Design review of the part built by this model. Coordinates are the model's own, in mm. A direction names the side the tool comes from. Coordinates: 2 decimals unless noted, no trailing zeros. Write each loop counter-clockwise with the first axis right and the second up, starting at its lowest first coordinate (ties: lowest second). Pieces come first, ordered by that corner, then holes. Notation, with made-up numbers: (55.5, 13) - (60.5, 13) arc R19 cw to (60.5, 46) - close; hole circle Ø11 at (86.25, 11). An arc over 180 degrees is marked (long way). Use a Markdown table: item, result.
from build123d import *

# Parameters (mm, degrees)
SKETCH1_R           = 7
SKETCH1_R_2         = 2.75
BOSS_EXTRUDE1_DEPTH = 7
SKETCH2_R           = 8
SKETCH2_R_2         = 6
BOSS_EXTRUDE2_DEPTH = 17
FILLET1_R           = 3
FILLET2_R           = 3
SKETCH3_R           = 1


with BuildPart() as part:
    # Sketch1 → Boss-Extrude1 (new body)
    with BuildSketch(Plane(origin=(0, 0, 0), x_dir=(1, 0, 0), z_dir=(0, 1, 0))):
        with BuildLine():
            ThreePointArc((-15.634333704, 6.748663161), (-22.25, 0), (-15.634333704, -6.748663161))
            ThreePointArc((-15.634333704, -6.748663161), (-12.054001616, -7.488359295), (-8.978814065, -9.465516285))
            ThreePointArc((-8.978814065, -9.465516285), (-0.068820662, -12.999999969), (8.841661443, -9.466748488))
            ThreePointArc((8.841661443, -9.466748488), (11.954703039, -7.474770851), (15.578657445, -6.749541689))
            ThreePointArc((15.578657445, -6.749541689), (22.25, 0), (15.578657445, 6.749541689))
            ThreePointArc((15.578657445, 6.749541689), (11.954703039, 7.474770851), (8.841661443, 9.466748488))
            ThreePointArc((8.841661443, 9.466748488), (-0.068820662, 12.999999969), (-8.978814065, 9.465516285))
            ThreePointArc((-8.978814065, 9.465516285), (-12.054001616, 7.488359295), (-15.634333704, 6.748663161))
        make_face()
        with Locations(Location((0, 0, 0), (0, 0, 270))):
            Circle(SKETCH1_R, mode=Mode.SUBTRACT)
        with Locations(Location((-15.5, 0, 0), (0, 0, 270))):
            Circle(SKETCH1_R_2, mode=Mode.SUBTRACT)
        with Locations(Location((15.5, 0, 0), (0, 0, 270))):
            Circle(SKETCH1_R_2, mode=Mode.SUBTRACT)
    extrude(amount=BOSS_EXTRUDE1_DEPTH)

    # Sketch2 → Boss-Extrude2 (add)
    with BuildSketch(Plane(origin=(0, 7, 0), x_dir=(1, 0, 0), z_dir=(0, 1, 0))):
        with Locations(Location((0, 0, 0), (0, 0, 270))):
            Circle(SKETCH2_R)
        with Locations(Location((0, 0, 0), (0, 0, 270))):
            Circle(SKETCH2_R_2, mode=Mode.SUBTRACT)
    extrude(amount=BOSS_EXTRUDE2_DEPTH)

    # Fillet1
    # the kernel refuses this fillet: 3 mm, written as the material it adds along each edge
    with BuildSketch(Plane(origin=(0, 7, 0), x_dir=(0, 0, 1), z_dir=(-1, 0, 0))) as fillet1_piece_1:
        with BuildLine():
            CenterArc((4, -2.236067977), FILLET1_R, 0, 48.189685104)
            Line((6, 0), (6.04, 0.04472136))
            ThreePointArc((6.04, 0.04472136), (6.5, 0.06), (7, 0.06))
            Line((7, 0.06), (7.06, 0))
            Line((7.06, 0), (7.06, -2.236067977))
            Line((7.06, -2.236067977), (7, -2.236067977))
        make_face()
    revolve(axis=Axis((0, 7, 0), (0, 1, 0)))
    with BuildSketch(Plane(origin=(0, 7, 0), x_dir=(0, 0, 1), z_dir=(-1, 0, 0))) as fillet1_piece_2:
        with BuildLine():
            CenterArc((8 + FILLET1_R, FILLET1_R), FILLET1_R, 180, 90)
            Line((8, FILLET1_R), (8 - FILLET1_R * 0.02, FILLET1_R))
            Line((8 - FILLET1_R * 0.02, FILLET1_R), (8 - FILLET1_R * 0.02, -FILLET1_R * 0.02))
            Line((8 - FILLET1_R * 0.02, -FILLET1_R * 0.02), (8 + FILLET1_R, -FILLET1_R * 0.02))
            Line((8 + FILLET1_R, -FILLET1_R * 0.02), (8 + FILLET1_R, 0))
        make_face()
    revolve(axis=Axis((0, 7, 0), (0, 1, 0)))

    # Fillet2
    fillet2_edges = [part.edges().sort_by_distance(p)[0] for p in [
        (0, 7, -6),
    ]]
    fillet(fillet2_edges, radius=FILLET2_R)


with BuildPart() as body_2:
    # Sketch3 → Revolve1 (revolve)
    with BuildSketch(Plane(origin=(0, 0, 0), x_dir=(0, 0, -1), z_dir=(1, 0, 0))):
        with Locations((8.5, 19.608844607)):
            Circle(SKETCH3_R)
    revolve(axis=Axis((0, 0, 0), (0, 1, 0)))


with BuildPart() as part_1:
    add(part.part)

    # Intersect1: read off the stored shape, not the designer's step
    # Intersect1: cut body 2
    add(body_2.part, mode=Mode.SUBTRACT)


solid = part_1.part
(1) Take a section at A-A on y = 12. Write out the cut boundary in (x, z), and give its area (3 significant figures).
Determined:
| item | result |
|---|---|
| outline | circle Ø16 at (0, 0); hole circle Ø12 at (0, 0) |
| area | 88.0 mm2 |
(2) Take a section at C-C on x = 12. Write out the cut boundary in (y, z), and give its area (3 significant figures).
Determined:
| item | result |
|---|---|
| outline | (0, -7.46) - (7, -7.46) - (7, 7.46) - (0, 7.46) - close |
| area | 104 mm2 |
(3) For pin 1 (3.5 mm diameter, centred on x = 15.5, z = 0, fed in from +Y); pin 2 (10 mm diameter, centred on y = 12.5, z = -8.5, fed in from +X); pin 3 (1.5 mm diameter, centred on x = 16.5, y = 4, fed in from +Z); pin 4 (5 mm diameter, centred on x = -13, z = -2.5, fed in from +Y), all flat-tipped, find the tip position at first contact; note any pin that passes through.
Determined:
| item | result |
|---|---|
| pin 1 | through |
| pin 2 | x = 7.19 |
| pin 3 | z = 6.75 |
| pin 4 | y = 7.01 |
(4) For L1, parallel to X at y = 1.5, z = 0; L2, parallel to X at y = 16.25, z = 0; L3, parallel to Y at x = 9, z = 8.75, list the stretches that pass through material, from the lowest coordinate up. Write a range as from..to.
Determined:
| item | result |
|---|---|
| L1 | -22.25..-18.25, -12.75..-7, 7..12.75, 18.25..22.25 |
| L2 | -8..-6, 6..8 |
| L3 | 0..7 |
(5) Draft analysis for pull direction X (two halves, no side actions). For faces 4 (the cylindrical face through (18.227, 3.451, -0.358)), 5 (the flat face through (5, 0, 6)), 6 (the cylindrical face through (0, 3, 13)), state which applies: +X half, -X half, draft (parallel to the pull), parting line (faces both ways), or undercut.
Determined:
| item | result |
|---|---|
| face 4 | undercut |
| face 5 | draft |
| face 6 | parting line |
(6) Machinability: for faces 1 (the cylindrical face through (-7.81, 22.21, -1.73)), 2 (the cylindrical face through (-2.3, 15.93, 5.54)), 3 (the cylindrical face through (-6.834, 2.349, -1.517)), which of the approach directions +Z, -Z, +X, -X, +Y, -Y give a long, thin tool a straight path to every point of the face, cutting with its end or side? Answer none if there is none.
Determined:
| item | result |
|---|---|
| face 1 | +Y |
| face 2 | +Y, -Y |
| face 3 | -Y |
(7) Take a section at B-B on z = 0. State how many separate pieces and enclosed holes the cut face has, and give its area (3 significant figures).
Determined:
| item | result |
|---|---|
| separate pieces | 4 |
| enclosed holes | 0 |
| area | 208 mm2 |
